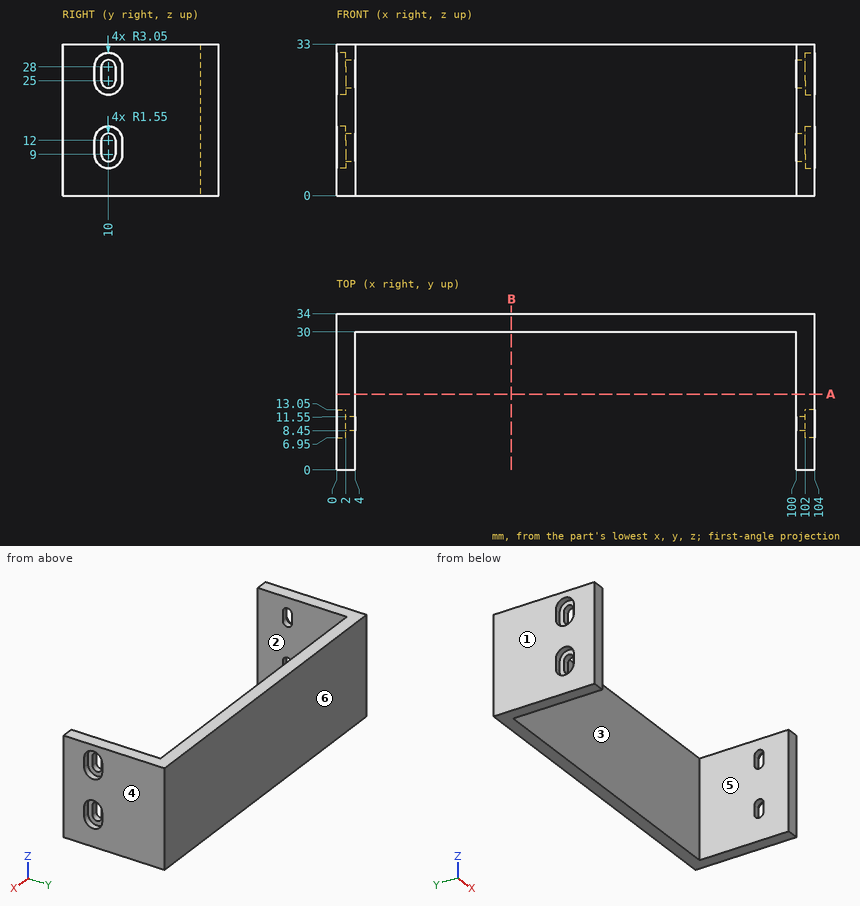
Geometry: see drawing. Coordinates: mm, zero at the bounding-box minimum. A direction names the side the tool comes from. Round coordinates to 2 decimals unless told otherwise and drop trailing zeros. Order: outer loops, then holes, each group sorted by start corner. A loop starts at its lowest first (then second) coordinate and runs counter-clockwise, first axis right, second up. Notation, with made-up numbers: (54.5, 76) - (96.5, 76) arc R18 ccw to (96.5, 104) - close; hole circle Ø9 at (-38, 57.25). An arc over 180 degrees is marked (long way). Use a Markdown table: item, result. Add a question column.
1. Section query A-A (y = 16.5). Return the cut outline in (x, z), then the cut area to 3 significant figures.
2. Section query B-B (x = 38). Return the cut outline in (y, z), then the cut area to 3 significant figures.
3. First-contact query: pin 1 (1.8 mm diameter, centred on y = 11.5, z = 28, fed in from +X); pin 2 (1 mm diameter, centred on x = 20.5, z = 25, fed in from -Y); pin 3 (3 mm diameter, centred on y = 8.5, z = 9, fed in from -X). Flat tips, straight axial feed; report the tip coordinate or a pass-through.
4. Mould query, pull axis X, two halves, no side actions, for the marked faces 3, 4, 5 and 6. Classes: +X half, -X half, draft (parallel to the pull), parting line (faces both ways), or undercut.
5. Line query: probe 1 along X at (y, z) = (15.5, 11.5); probe 2 along Y at (x, z) = (39, 14.5). Output: solid intervals per line, ascending.
6. Set-up query: the marked faces 1 and 2. Return all of +Z, -Z, +X, -X, +Y, -Y with unobstructed straight access to the full face (end or side cutting, diameter ignored); none if empty.
Derived:
| question | item | result |
|---|---|---|
| 1 | outline | (0, 0) - (4, 0) - (4, 33) - (0, 33) - close; (100, 0) - (104, 0) - (104, 33) - (100, 33) - close |
| 1 | area | 264 mm2 |
| 2 | outline | (30, 0) - (34, 0) - (34, 33) - (30, 33) - close |
| 2 | area | 132 mm2 |
| 3 | pin 1 | x = 102 |
| 3 | pin 2 | y = 30 |
| 3 | pin 3 | x = 2 |
| 4 | face 3 | undercut |
| 4 | face 4 | +X half |
| 4 | face 5 | undercut |
| 4 | face 6 | draft |
| 5 | probe 1 | 0 to 4, 100 to 104 |
| 5 | probe 2 | 30 to 34 |
| 6 | face 1 | +Z, -Z, -X, +Y, -Y |
| 6 | face 2 | +Z, -Z, -Y |
